```python
from build123d import *

# Parameters (mm, degrees)
SKETCH1_W                               = 304.8
SKETCH1_H                               = 304.8
BOSS_EXTRUDE1_DEPTH                     = 38.1
SKETCH2_R                               = 6.5151
HAAS_T_SLOT_HOLES_DEPTH                 = 219.867836833
SKETCH3_R                               = 9.779
HAAS_COUNTER_BORES_DEPTH                = 22.225
SKETCH4_R                               = 6.5151
TORMACH_T_SLOT_HOLES_DEPTH              = 219.867836833
SKETCH5_R                               = 9.779
TORMACH_COUNTER_BORES_DEPTH             = 22.225
SKETCH6_R                               = 3.0734
SPROCKET_LOCATING_HOLES_DEPTH           = 6.35
SKETCH7_R                               = 3.175
SPROCKET_MOUNTING_CLEARANCE_HOLES_DEPTH = 9.525
SKETCH8_R                               = 5.9182
F_1_2_13_TAPPED_HOLES_DEPTH             = 19.05


with BuildPart() as part:
    # Sketch1 → Boss-Extrude1 (new body)
    with BuildSketch(Plane.XY):
        Rectangle(SKETCH1_W, SKETCH1_H)
    extrude(amount=BOSS_EXTRUDE1_DEPTH)

    # Sketch2 → HAAS T-Slot Holes (cut, through all)
    with BuildSketch(Plane.XY.offset(38.1)):
        with Locations((-127, 101.6)):
            Circle(SKETCH2_R)
        with Locations((127, 101.6)):
            Circle(SKETCH2_R)
        with Locations((127, -101.6)):
            Circle(SKETCH2_R)
        with Locations((-127, -101.6)):
            Circle(SKETCH2_R)
        Circle(SKETCH2_R)
    extrude(amount=-HAAS_T_SLOT_HOLES_DEPTH, mode=Mode.SUBTRACT)

    # Sketch3 → HAAS Counter Bores (cut)
    with BuildSketch(Plane.XY.offset(38.1)):
        with Locations((-127, 101.6)):
            Circle(SKETCH3_R)
        with Locations((127, 101.6)):
            Circle(SKETCH3_R)
        Circle(SKETCH3_R)
        with Locations((127, -101.6)):
            Circle(SKETCH3_R)
        with Locations((-127, -101.6)):
            Circle(SKETCH3_R)
    extrude(amount=-HAAS_COUNTER_BORES_DEPTH, mode=Mode.SUBTRACT)

    # Sketch4 → Tormach T-Slot Holes (cut, through all)
    with BuildSketch(Plane.XY.offset(38.1)):
        with Locations((-101.6, 90.4875)):
            Circle(SKETCH4_R)
        with Locations((101.6, 90.4875)):
            Circle(SKETCH4_R)
        with Locations((-101.6, -90.4875)):
            Circle(SKETCH4_R)
        with Locations((101.6, -90.4875)):
            Circle(SKETCH4_R)
    extrude(amount=-TORMACH_T_SLOT_HOLES_DEPTH, mode=Mode.SUBTRACT)

    # Sketch5 → Tormach Counter bores (cut)
    with BuildSketch(Plane.XY.offset(38.1)):
        with Locations((-101.6, 90.4875)):
            Circle(SKETCH5_R)
        with Locations((101.6, 90.4875)):
            Circle(SKETCH5_R)
        with Locations((101.6, -90.4875)):
            Circle(SKETCH5_R)
        with Locations((-101.6, -90.4875)):
            Circle(SKETCH5_R)
    extrude(amount=-TORMACH_COUNTER_BORES_DEPTH, mode=Mode.SUBTRACT)

    # Sketch6 → Sprocket Locating Holes (cut)
    with BuildSketch(Plane.XY.offset(38.1)):
        with Locations((0, 43.50004)):
            Circle(SKETCH6_R)
        with Locations((0, -43.50004)):
            Circle(SKETCH6_R)
    extrude(amount=-SPROCKET_LOCATING_HOLES_DEPTH, mode=Mode.SUBTRACT)

    # Sketch7 → Sprocket Mounting clearance holes (cut)
    with BuildSketch(Plane.XY.offset(38.1)):
        with Locations((43.50004, 0)):
            Circle(SKETCH7_R)
        with Locations((37.672139706, -21.75002)):
            Circle(SKETCH7_R)
        with Locations((21.75002, -37.672139706)):
            Circle(SKETCH7_R)
        with Locations((-21.75002, -37.672139706)):
            Circle(SKETCH7_R)
        with Locations((-37.672139706, -21.75002)):
            Circle(SKETCH7_R)
        with Locations((-43.50004, 0)):
            Circle(SKETCH7_R)
        with Locations((-37.672139706, 21.75002)):
            Circle(SKETCH7_R)
        with Locations((-21.75002, 37.672139706)):
            Circle(SKETCH7_R)
        with Locations((21.75002, 37.672139706)):
            Circle(SKETCH7_R)
        with Locations((37.672139706, 21.75002)):
            Circle(SKETCH7_R)
    extrude(amount=-SPROCKET_MOUNTING_CLEARANCE_HOLES_DEPTH, mode=Mode.SUBTRACT)

    # Sketch8 → 1/2-13 Tapped Holes (cut)
    with BuildSketch(Plane.XY.offset(38.1)):
        with Locations((-71.4375, 106.4641)):
            Circle(SKETCH8_R)
        with Locations((71.4375, 106.4641)):
            Circle(SKETCH8_R)
        with Locations((71.4375, -106.4641)):
            Circle(SKETCH8_R)
        with Locations((-71.4375, -106.4641)):
            Circle(SKETCH8_R)
    extrude(amount=-F_1_2_13_TAPPED_HOLES_DEPTH, mode=Mode.SUBTRACT)


solid = part.part
```
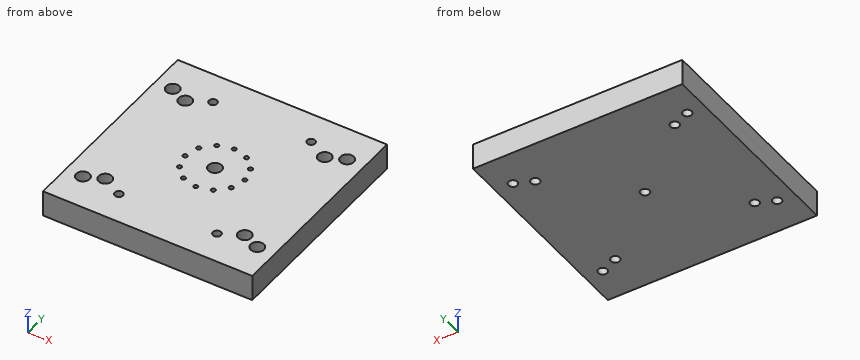
Here's how the part is built. I have some questions about the finished solid (model axes, mm). Give positions to 0.01 mm unless a question says otherwise; leave off trailing zeros. Write each loop counter-clockwise with the first axis right and the second up, starting at its lowest first coordinate (ties: lowest second). Pieces come first, ordered by that corner, then holes.
(1) Will these pins go through, and if not, where does the flat tip stop? pin 1 (3 mm diameter, centred on x = -22.5, y = 37.5, fed in from +Z) (3 decimals); pin 2 (10.5 mm diameter, centred on x = 0, y = 0, fed in from +Z).
Output values:
pin 1: stops at z = 28.575
pin 2: passes through
(2) If I drill on L1, parallel to Y at x = -101.6, z = 29.25; L2, parallel to Y at x = -101.6, z = 11; L3, parallel to Y at x = 0, z = 9.5, over which ranges is the centre line in solid material (lowest first)?
Output values:
L1: y = -152.4 to -100.27, -80.71 to 80.71, 100.27 to 152.4
L2: y = -152.4 to -97, -83.97 to 83.97, 97 to 152.4
L3: y = -152.4 to -6.52, 6.52 to 152.4
(3) Imagine slicing it at A-A, the plane x = 127. Write out the boundary of the cut face in (y, z) (3 decimals).
Output values:
outline: (-152.4, 0) - (-108.115, 0) - (-108.115, 15.875) - (-111.379, 15.875) - (-111.379, 38.1) - (-152.4, 38.1) - close; (-95.085, 0) - (95.085, 0) - (95.085, 15.875) - (91.821, 15.875) - (91.821, 38.1) - (-91.821, 38.1) - (-91.821, 15.875) - (-95.085, 15.875) - close; (108.115, 0) - (152.4, 0) - (152.4, 38.1) - (111.379, 38.1) - (111.379, 15.875) - (108.115, 15.875) - close
